```python
from build123d import *

# Parameters (mm, degrees)
F1_W     = 2
F1_H     = 150
F5_DEPTH = 2
F7_DEPTH = 2


# Not quite as in the source:
# - the program builds the solid bodies; features that only make, move or delete a surface that nothing else refers to are left out


with BuildPart() as f4:
    # F1 (on Front) → F4 (revolve)
    with BuildSketch(Plane.XZ):
        with Locations((-1, -7.0591911674)):
            Rectangle(F1_W, F1_H)
    revolve(axis=Axis((0, 0, 16.0941202193), (0, 0, -1)))

    # F0 (on Front) → F5 (join)
    with BuildSketch(Plane.XZ):
        with BuildLine():
            Line((0, 63.3778050542), (0, -29.2516257614))
            Line((0, -29.2516257614), (54.3039664626, -29.2516257614))
            add(Edge.make_bspline(
                [(0, 63.3778050542), (16.6847622445, 40.4423802167), (44.0846316514, 2.7776154372), (51.4310467474, -20.2473764435), (54.3039664626, -29.2516257614)],
                knots=[0, 0, 0, 0, 0.6089358309, 1, 1, 1, 1], degree=3))
        make_face()
    extrude(amount=F5_DEPTH)

    # F2 (on Front) → F7 (join)
    with BuildSketch(Plane.XZ):
        Polygon((0.1667886972, -30.2148442715), (0, 56.7073263228), (-39.3750006333, -30.2148442715), align=None)
    extrude(amount=F7_DEPTH)


solid = f4.part
```
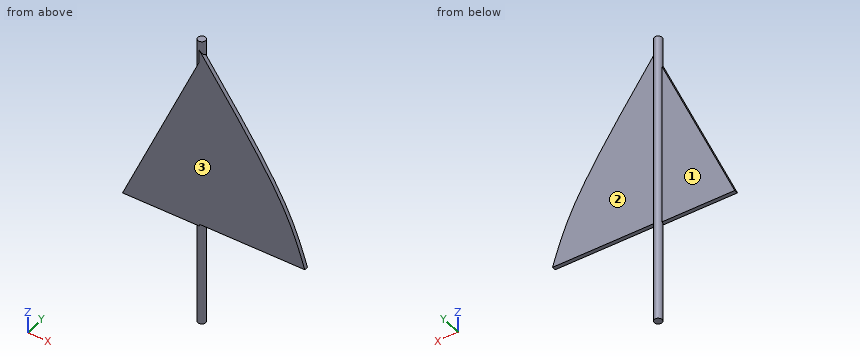
The listing builds one solid part. Answer for the finished solid, in the listing's coordinates (mm). Face numbers are marked on the shaded views. A direction names the side the tool comes from. Round coordinates to 2 decimals unless told otherwise and drop trailing zeros. Loops run counter-clockwise (first coordinate to the right, second up) from the corner with the lowest first, then second, coordinate; pieces in that order, holes last.
Q1. Section A-A, the plane z = -45 is taken. Determine the outline of the cut face in (x, y).
Q2. Which of the six approach directions +Z, -Z, +X, -X, +Y, -Y give full straight-line access (tool end or side, diameter ignored) to the marked faces 1, 2 and 3?
Q3. Section B-B, the plane y = 1.1 is taken. Determine the outline of the cut face in (x, z).
Q4. Given pin 1 Ø2 at (x, y) = (38, -1) entering from -Z; pin 2 Ø1 at (y, z) = (0, -31) entering from +X; pin 3 Ø8 at (x, z) = (41, -27.5) entering from +Y, each flat-ended and moving along its own axis, determine where each tip first touches the part or whether it passes through.
Q5. Section C-C, the plane x = -29 is taken. Determine the outline of the cut face in (y, z), then the cut area to 3 significant figures.
Q6. Find the intervals of material crossed by line 1 (Y direction, x = 47, z = -27.5); line 2 (X direction, y = 0.1, z = 26.5); line 3 (Z direction, x = -2, y = -1.65), in increasing order.
Completed:
1. outline: circle Ø4 at (0, 0)
2. face 1: +Z, -Z, -X, +Y
2. face 2: +Z, -Z, +X, +Y
2. face 3: +Z, -Z, +X, -X, -Y
3. outline: (-1.67, -82.06) - (1.67, -82.06) - (1.67, 67.94) - (-1.67, 67.94) - close
4. pin 1: stops at z = -29.25
4. pin 2: stops at x = 2
4. pin 3: stops at y = 0
5. outline: (-2, -30.21) - (0, -30.21) - (0, -7.31) - (-2, -7.31) - close
5. area: 45.8 mm2
6. line 1: y = -2 to 0
6. line 2: x = -2 to 2
6. line 3: z = -30.21 to 52.29
